Geometry: final body of the model. Coordinates: model frame, mm. Face numbers are marked on the shaded views. Round coordinates to 2 decimals unless told otherwise and drop trailing zeros. Write each loop counter-clockwise with the first axis right and the second up, starting at its lowest first coordinate (ties: lowest second). Pieces come first, ordered by that corner, then holes. Notation, with made-up numbers: M 27.5,-2.75 L 57.5,-2.75 A23 ccw 57.5,34.25 Z; hole C -11,-18.5 d5. An arc over 180 degrees is marked long. Answer as CSV lines item,"result". Start each with the question number.
Q1. Ray query, probe 1 along X at (y, z) = (0, 3) (3 decimals); probe 2 along Y at (x, z) = (-28.5, 0.75); probe 3 along X at (y, z) = (0, 2.5) (3 decimals). Return the intervals inside material, ascending.
Q2. Section query C-C on z = 2.25. Output: boundary loops of the cut face in (x, y) (3 decimals).
Q3. Section query A-A on x = 0. Output: boundary loops of the cut face in (y, z) (3 decimals), and give its area (3 significant figures).
Q4. Section query B-B on y = 0. Output: boundary loops of the cut face in (x, z) (3 decimals).
Q5. Mould query, pull axis X, two halves, no side actions, for the marked faces 1, 2 and 3. Classes: pulls with the +X half, pulls with the -X half, needs draft (parallel to the pull), parting line crosses it, or undercut.
Q6. First-contact query: pin 1 (2 mm diameter, centred on y = 12.5, z = 2, fed in from -X); pin 2 (1.5 mm diameter, centred on x = 17.5, z = 3.5, fed in from +Y); pin 3 (3 mm diameter, centred on x = 29, z = 1.5, fed in from +Y). Flat tips, straight axial feed; report the tip coordinate or a pass-through.
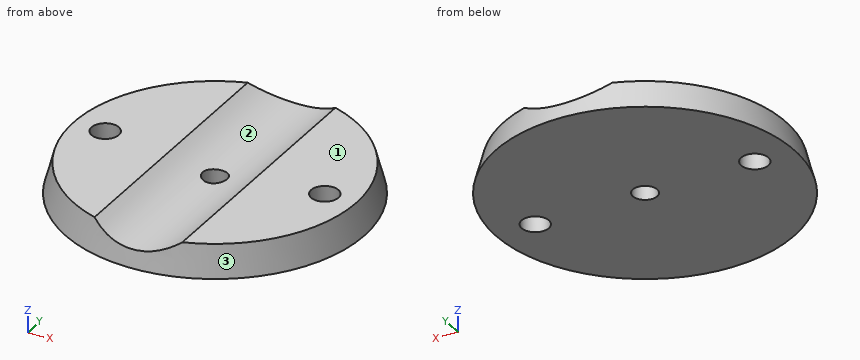
```python
from build123d import *

# Parameters (mm, degrees)
F3_DEPTH      = 38.9011
F3_DEPTH_BACK = 38.9011
F4_R          = 3.175
F4_R_2        = 3.5687
F5_DEPTH      = 7.9512001


with BuildPart() as f1:
    # F0 (on Front) → F1 (revolve)
    with BuildSketch(Plane.XZ):
        Polygon((36.7698503303, 7.9502), (0, 7.9502), (0, 0), (38.9001, 0), align=None)
    revolve(axis=Axis((0, 0, 3.9751), (0, 0, -1)))

    # F2 (on Front) → F3 (cut, two sides)
    with BuildSketch(Plane.XZ) as f3_sk:
        with BuildLine():
            Line((11.4236482351, 7.9502), (-11.4236482351, 7.9502))
            ThreePointArc((-11.4236482351, 7.9502), (0, 4.2672), (11.4236482351, 7.9502))
        make_face()
    extrude(amount=-F3_DEPTH, mode=Mode.SUBTRACT)
    extrude(f3_sk.sketch, amount=F3_DEPTH_BACK, mode=Mode.SUBTRACT)

    # F4 (on face) → F5 (cut, through all)
    with BuildSketch(Plane(origin=(0, 0, 0), x_dir=(1, 0, 0), z_dir=(0, 0, -1))):
        Circle(F4_R)
        with Locations((-28.575, 0)):
            Circle(F4_R_2)
        with Locations((28.575, 0)):
            Circle(F4_R_2)
    extrude(amount=-F5_DEPTH, mode=Mode.SUBTRACT)


solid = f1.part
```
Entries:
1,probe 1,"x = -38.096 to -32.144, -25.006 to -3.175, 3.175 to 25.006, 32.144 to 38.096"
1,probe 2,"y = -26.18 to -3.57, 3.57 to 26.18"
1,probe 3,"x = -38.23 to -32.144, -25.006 to -3.175, 3.175 to 25.006, 32.144 to 38.23"
2,outline,"C 0,0 d76.594; hole C -28.575,0 d7.137; hole C 0,0 d6.35; hole C 28.575,0 d7.137"
3,outline,"M -38.9,0 L -3.175,0 L -3.175,4.267 L -37.757,4.267 Z; M 3.175,0 L 38.9,0 L 37.757,4.267 L 3.175,4.267 Z"
3,area,"300 mm^2"
4,outline,"M -38.9,0 L -32.144,0 L -32.144,7.95 L -36.77,7.95 Z; M -25.006,0 L -3.175,0 L -3.175,4.527 A19.558 cw -11.424,7.95 L -25.006,7.95 Z; M 3.175,0 L 25.006,0 L 25.006,7.95 L 11.424,7.95 A19.558 cw 3.175,4.527 Z; M 32.144,0 L 38.9,0 L 36.77,7.95 L 32.144,7.95 Z"
5,face 1,"needs draft"
5,face 2,"undercut"
5,face 3,"parting line crosses it"
6,pin 1,"stops at x = -36.71"
6,pin 2,"stops at y = 34.13"
6,pin 3,"stops at y = 27.05"
